The listing builds one solid part. Answer for the finished solid, in the listing's coordinates (mm). Round coordinates to 2 decimals unless told otherwise and drop trailing zeros. Order: outer loops, then holes, each group sorted by start corner. A loop starts at its lowest first (then second) coordinate and runs counter-clockwise, first axis right, second up. Notation, with made-up numbers: M 34,26 L 87,26 A14 cw 87,39 Z; hole C 82.5,14.25 d9. An arc over 180 degrees is marked long. Write item = value, one per line. Start each with the question number.
(1) A cutting plane is placed at B-B, the plane y = -65. Determine the outline of the cut face in (x, z) (3 decimals).
(2) A cutting plane is placed at D-D, the plane x = 5. Determine the outline of the cut face in (y, z) (3 decimals), and give its area (3 significant figures).
(3) Straight lines are drawn through the part: probe 1 along X at (y, z) = (-42, 3.05); probe 2 along Y at (x, z) = (36, 1.85); probe 3 along X at (y, z) = (-65.5, 0.6) (3 decimals). For each, find the intervals that lie inside material, in ascending order. Write a range as from..to.
(4) A cutting plane is placed at A-A, the plane y = 20.32. Determine the outline of the cut face in (x, z) (3 decimals).
(5) Each of these flat-tipped pins is pushed along its axis until it touches: pin 1 (1.3 mm diameter, centred on y = -41, z = 1.5, fed in from +X); pin 2 (2.5 mm diameter, centred on x = 78.56, y = -32.65, fed in from -Z); pin 3 (6 mm diameter, centred on x = 72.5, y = -40, fed in from -Z); pin 4 (1 mm diameter, centred on y = 18.5, z = 2, fed in from -X). Where does it stop, or does it pass through?
(6) A cutting plane is placed at C-C, the plane z = 1.35. Count the separate pieces of the cut face and the enclosed holes in it, and give its area (3 significant figures).
from build123d import *

# Parameters (mm, degrees)
SKETCH1_R           = 1.524
BOSS_EXTRUDE1_DEPTH = 3.175


with BuildPart() as part:
    # Sketch1 → Boss-Extrude1 (new body)
    with BuildSketch(Plane.XY):
        with BuildLine():
            Line((0.762, 0), (21.9075, 0))
            Line((21.9075, 0), (21.9075, -34.42335))
            ThreePointArc((21.9075, -34.42335), (22.465461582, -35.770388418), (23.8125, -36.32835))
            Line((23.8125, -36.32835), (31.75, -36.32835))
            Line((31.75, -36.32835), (31.75, -71.25335))
            ThreePointArc((31.75, -71.25335), (32.307961582, -72.600388418), (33.655, -73.15835))
            Line((33.655, -73.15835), (70.485, -73.15835))
            ThreePointArc((70.485, -73.15835), (71.832038418, -72.600388418), (72.39, -71.25335))
            Line((72.39, -71.25335), (72.39, -36.32835))
            Line((72.39, -36.32835), (80.3275, -36.32835))
            ThreePointArc((80.3275, -36.32835), (81.674538418, -35.770388418), (82.2325, -34.42335))
            Line((82.2325, -34.42335), (82.2325, 0))
            Line((82.2325, 0), (103.378, 0))
            ThreePointArc((103.378, 0), (103.916815367, 0.223184633), (104.14, 0.762))
            Line((104.14, 0.762), (104.14, 5.08))
            Line((104.14, 5.08), (117.348, 5.08))
            ThreePointArc((117.348, 5.08), (117.886815367, 5.303184633), (118.11, 5.842))
            Line((118.11, 5.842), (118.11, 10.668))
            ThreePointArc((118.11, 10.668), (117.886815367, 11.206815367), (117.348, 11.43))
            Line((117.348, 11.43), (104.14, 11.43))
            Line((104.14, 11.43), (104.14, 24.638))
            ThreePointArc((104.14, 24.638), (103.916815367, 25.176815367), (103.378, 25.4))
            Line((103.378, 25.4), (0.762, 25.4))
            ThreePointArc((0.762, 25.4), (0.223184633, 25.176815367), (0, 24.638))
            Line((0, 24.638), (0, 11.43))
            Line((0, 11.43), (-13.208, 11.43))
            ThreePointArc((-13.208, 11.43), (-13.746815367, 11.206815367), (-13.97, 10.668))
            Line((-13.97, 10.668), (-13.97, 5.842))
            ThreePointArc((-13.97, 5.842), (-13.746815367, 5.303184633), (-13.208, 5.08))
            Line((-13.208, 5.08), (0, 5.08))
            Line((0, 5.08), (0, 0.762))
            ThreePointArc((0, 0.762), (0.223184633, 0.223184633), (0.762, 0))
        make_face()
        with Locations((25.58415, 20.32)):
            Circle(SKETCH1_R, mode=Mode.SUBTRACT)
        with Locations((78.55585, 20.32)):
            Circle(SKETCH1_R, mode=Mode.SUBTRACT)
        with Locations((78.55585, -32.6517)):
            Circle(SKETCH1_R, mode=Mode.SUBTRACT)
        with Locations((25.58415, -32.6517)):
            Circle(SKETCH1_R, mode=Mode.SUBTRACT)
        with BuildLine():
            Line((38.7985, -40.13835), (38.7985, -42.67835))
            ThreePointArc((38.7985, -42.67835), (36.195, -45.28185), (33.5915, -42.67835))
            Line((33.5915, -42.67835), (33.5915, -40.13835))
            ThreePointArc((33.5915, -40.13835), (36.195, -37.53485), (38.7985, -40.13835))
        make_face(mode=Mode.SUBTRACT)
        with BuildLine():
            Line((70.5485, -40.13835), (70.5485, -42.67835))
            ThreePointArc((70.5485, -42.67835), (67.945, -45.28185), (65.3415, -42.67835))
            Line((65.3415, -42.67835), (65.3415, -40.13835))
            ThreePointArc((65.3415, -40.13835), (67.945, -37.53485), (70.5485, -40.13835))
        make_face(mode=Mode.SUBTRACT)
        with BuildLine():
            Line((69.595, -63.63335), (69.595, -69.98335))
            ThreePointArc((69.595, -69.98335), (67.945, -71.63335), (66.295, -69.98335))
            Line((66.295, -69.98335), (66.295, -63.63335))
            ThreePointArc((66.295, -63.63335), (67.945, -61.98335), (69.595, -63.63335))
        make_face(mode=Mode.SUBTRACT)
        with BuildLine():
            Line((37.845, -63.63335), (37.845, -69.98335))
            ThreePointArc((37.845, -69.98335), (36.195, -71.63335), (34.545, -69.98335))
            Line((34.545, -69.98335), (34.545, -63.63335))
            ThreePointArc((34.545, -63.63335), (36.195, -61.98335), (37.845, -63.63335))
        make_face(mode=Mode.SUBTRACT)
    extrude(amount=BOSS_EXTRUDE1_DEPTH)


solid = part.part
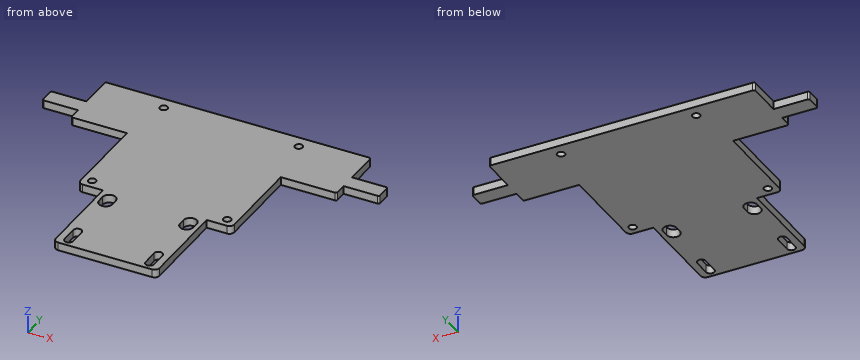
Reported:
q1.outline = M 31.75,0 L 34.545,0 L 34.545,3.175 L 31.75,3.175 Z; M 37.845,0 L 66.295,0 L 66.295,3.175 L 37.845,3.175 Z; M 69.595,0 L 72.39,0 L 72.39,3.175 L 69.595,3.175 Z
q2.outline = M 0,0 L 25.4,0 L 25.4,3.175 L 0,3.175 Z
q2.area = 80.6 mm²
q3.probe_1 = 31.75..33.59, 38.8..65.34, 70.55..72.39
q3.probe_2 = -73.16..-71.62, -61.99..-45.27, -37.54..25.4
q3.probe_3 = 31.75..34.545, 37.845..66.295, 69.595..72.39
q4.outline = M 0,0 L 24.06,0 L 24.06,3.175 L 0,3.175 Z; M 27.108,0 L 77.032,0 L 77.032,3.175 L 27.108,3.175 Z; M 80.08,0 L 104.14,0 L 104.14,3.175 L 80.08,3.175 Z
q5.pin_1 = 72.39
q5.pin_2 = through
q5.pin_3 = 0
q5.pin_4 = 0
q6.separate_pieces = 1
q6.enclosed_holes = 8
q6.area = 6,350 mm²
